Verification items for this drawing (mm, ordinates from the low corner). Coordinates: 2 decimals unless noted, no trailing zeros. Order: outer loops, then holes, each group sorted by start corner. A loop starts at its lowest first (then second) coordinate and runs counter-clockwise, first axis right, second up. Notation, with made-up numbers: M 25,89 L 34,89 A33 ccw 34,120 Z; hole C 41.5,20 d7. An arc over 180 degrees is marked long. Answer as a JSON object with one key per item and string values. Group by question number.
(1) Cross-section at B-B (z = 2.1). Enter the section's corners in (x, y), plus the area to 3 significant figures.
(2) Gauge pin test, flat ends, axial feed: pin 1 Ø1.5 at (x, y) = (31.5, 21) entering from +Z; pin 2 Ø2 at (x, y) = (59.89, 22) entering from -Z; pin 3 Ø0.8 at (x, z) = (57.5, 1) entering from -Y. Record the tip position at first contact, or that the pin passes through.
(3) Material ranges on line 1 (Y direction, x = 30, z = 1.9); line 2 (Y direction, x = 47, z = 1.5); line 3 (Y direction, x = 58.5, z = 0.6) (1 decimal), recorded low to high.
(4) Cross-section at A-A (x = 30). Enter the section's corners in (y, z).
(5) Cross-section at C-C (y = 2). Enter the section's corners in (x, z), plus the area to 3 significant figures.
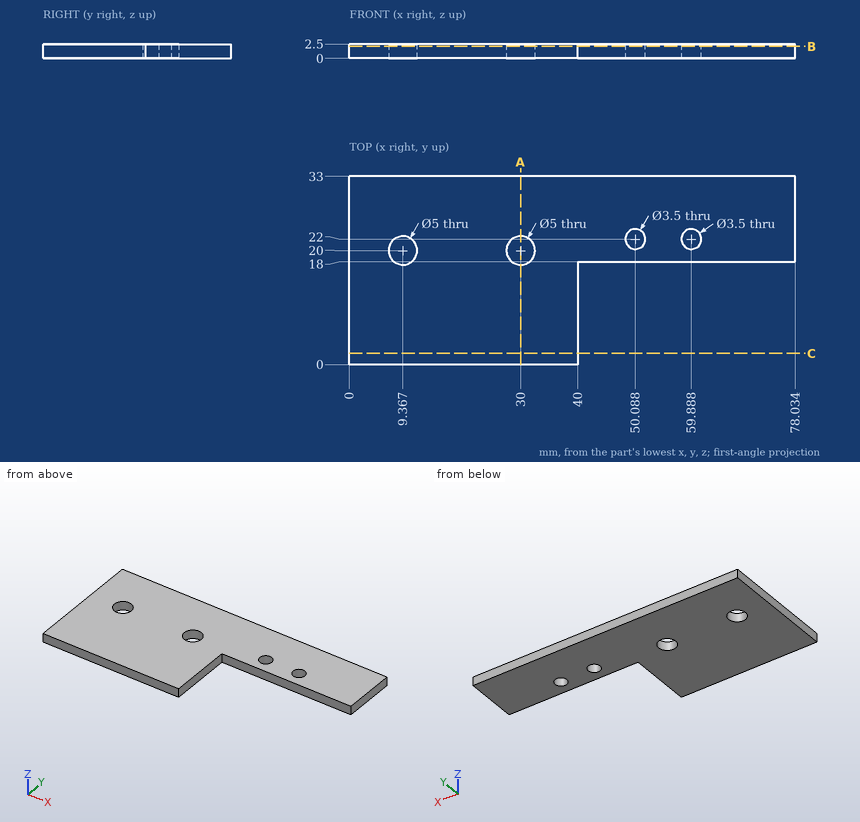
Taken from the geometry:
{
 "1": {"outline": "M 0,0 L 40,0 L 40,18 L 78.03,18 L 78.03,33 L 0,33 Z; hole C 9.37,20 d5; hole C 30,20 d5; hole C 50.09,22 d3.5; hole C 59.89,22 d3.5", "area": "1,830 mm²"},
 "2": {"pin 1": "stops at z = 2.5", "pin 2": "passes through", "pin 3": "stops at y = 18"},
 "3": {"line 1": "y = 0 to 17.5, 22.5 to 33", "line 2": "y = 18 to 33", "line 3": "y = 18 to 20.9, 23.1 to 33"},
 "4": {"outline": "M 0,0 L 17.5,0 L 17.5,2.5 L 0,2.5 Z; M 22.5,0 L 33,0 L 33,2.5 L 22.5,2.5 Z"},
 "5": {"outline": "M 0,0 L 40,0 L 40,2.5 L 0,2.5 Z", "area": "100 mm²"}
}
